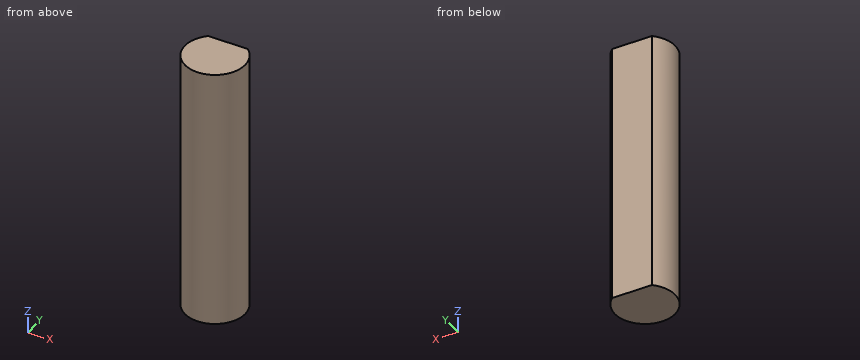
from build123d import *

# Parameters (mm, degrees)
SKETCH2_R                      = 4
BOSS_EXTRUDE1_DEPTH            = 35
CUT_EXTRUDE1_REACH             = 37
CUT_EXTRUDE1_DIRECTION_2_DEPTH = 1


with BuildPart() as part:
    # Sketch2 → Boss-Extrude1 (new body)
    with BuildSketch(Plane.XY):
        Circle(SKETCH2_R)
    extrude(amount=BOSS_EXTRUDE1_DEPTH)

    # Sketch3 → Cut-Extrude1 (cut, up to next)
    with BuildSketch(Plane.XY.offset(35), mode=Mode.PRIVATE) as cut_extrude1_sk1:
        with BuildLine():
            Line((-2.645751311, 3), (2.645751311, 3))
            ThreePointArc((2.645751311, 3), (0, 4), (-2.645751311, 3))
        make_face()
    cut_extrude1_tool1 = extrude(cut_extrude1_sk1.sketch, amount=-CUT_EXTRUDE1_REACH, mode=Mode.PRIVATE) & part.part
    add(cut_extrude1_tool1.solids().sort_by_distance((0, 3.404621, 35))[0], mode=Mode.SUBTRACT)

    # Sketch3 → Cut-Extrude1 direction 2 (cut)
    with BuildSketch(Plane.XY.offset(35)):
        with BuildLine():
            Line((-2.645751311, 3), (2.645751311, 3))
            ThreePointArc((2.645751311, 3), (0, 4), (-2.645751311, 3))
        make_face()
    extrude(amount=CUT_EXTRUDE1_DIRECTION_2_DEPTH, mode=Mode.SUBTRACT)


solid = part.part
The listing builds one solid part. Answer for the finished solid, in the listing's coordinates (mm). Give positions to 0.01 mm unless a question says otherwise; leave off trailing zeros. Order: outer loops, then holes, each group sorted by start corner. A loop starts at its lowest first (then second) coordinate and runs counter-clockwise, first axis right, second up. Notation, with made-up numbers: (0.25, 33) -> (16.25, 33) arc R7 cw to (16.25, 38) -> close; hole circle Ø3 at (-25, -14). An arc over 180 degrees is marked (long way). Put each result on its own line as item: value.
Item 1: A cutting plane is placed at B-B on y = -3.25. Give the vertices of the cut face in (x, z).
Established:
outline: (-2.33, 0) -> (2.33, 0) -> (2.33, 35) -> (-2.33, 35) -> close
Item 2: Given P1, Ø1.5, axis at y = 1.5, z = 28, coming from the +X side; P2, Ø1, axis at y = -2, z = 15, coming from the -X side, each flat-ended and moving along its own axis, determine where each tip first touches the part or whether it passes through.
Established:
P1: stops at x = 3.93
P2: stops at x = -3.71
Item 3: Straight lines are drawn through the part: line 1 (Y direction, x = -0.25, z = 7.5); line 2 (Y direction, x = 3, z = 8); line 3 (X direction, y = 2.5, z = 25). For each, find the intervals that lie inside material, in ascending order.
Established:
line 1: y = -3.99 to 3
line 2: y = -2.65 to 2.65
line 3: x = -3.12 to 3.12
Item 4: A cutting plane is placed at A-A on z = 33. Give the vertices of the cut face in (x, y), plus the area to 3 significant figures.
Established:
outline: (-2.65, 3) arc R4 ccw (long way) to (2.65, 3) -> close
area: 46.6 mm^2
